Build history of the part. All positions in model axes, mm. A direction names the side the tool comes from. Give positions to 0.01 mm unless a question says otherwise; leave off trailing zeros. Order: outer loops, then holes, each group sorted by start corner. A loop starts at its lowest first (then second) coordinate and runs counter-clockwise, first axis right, second up. Notation, with made-up numbers: (-11.75, 78) -> (27.25, 78) arc R19 ccw to (27.25, 86) -> close; hole circle Ø2 at (8, 0.25). An arc over 180 degrees is marked (long way). One line per item, written item: value. Start each with the question number.
(1) Pin check, flat tip, straight feed: pin 1 (15 mm diameter, centred on x = -41.5, z = -49, fed in from +Y). Stop position of the tip, or through.
(2) Which spindle directions (+Z, -Z, +X, -X, +Y, -Y) get a long thin tool onto all of the face, cutting with end or side? Do faces 5 (the flat face through (16, 0, -18)), 6 (the cylindrical face through (-26.452, 14.93, -40.881)). Say none if no direction does.
(3) Saw through at C-C on x = 14.5. Give the cut face in (y, z).
(4) Saw through at A-A on y = 15.5. Give the cut face in (x, z).
(5) Probe line 1 (X direction, y = 16, z = -45); line 2 (X direction, y = 14, z = 0); line 3 (Z direction, x = 60.5, y = 13.5). List the from-to ranges inside material, lowest first.
(6) Two-plate mould, pull along X, no slides. Class faces 1 (the flat face through (-70, 10, -70)), 2 (the flat face through (75, 10, 1)), 3 (the flat face through (-1, 10, 28)), 4 (the flat face through (-68, 20, -1)): +X half, -X half, draft (parallel to the pull), parting line (faces both ways), or undercut.
(7) Saw through at B-B on z = -16. Give the cut face in (x, y), plus the area to 3 significant figures.
(8) Saw through at D-D on y = 4.5. Give the cut face in (x, z), plus the area to 3 significant figures.
```python
from build123d import *

# Parameters (mm, degrees)
SKETCH1_W           = 150
SKETCH1_H           = 150
SKETCH1_W_2         = 130
SKETCH1_H_2         = 130
BOSS_EXTRUDE2_DEPTH = 20
SKETCH1_4_W         = 130
SKETCH1_4_H         = 130
BOSS_EXTRUDE3_DEPTH = 10
CHAMFER1_SIZE       = 10
SKETCH2_R           = 20
CUT_EXTRUDE2_DEPTH  = 10
BOSS_EXTRUDE4_START = 10
SKETCH3_R           = 25
SKETCH3_R_2         = 20
BOSS_EXTRUDE4_DEPTH = 10
SKETCH4_R           = 19
SKETCH4_R_2         = 15
BOSS_EXTRUDE5_DEPTH = 10


with BuildPart() as part:
    # Sketch1 → Boss-Extrude2 (new body)
    with BuildSketch(Plane(origin=(0, 0, 0), x_dir=(1, 0, 0), z_dir=(0, 1, 0))):
        Rectangle(SKETCH1_W, SKETCH1_H)
        Rectangle(SKETCH1_W_2, SKETCH1_H_2, mode=Mode.SUBTRACT)
    extrude(amount=BOSS_EXTRUDE2_DEPTH)

    # Sketch1<4> → Boss-Extrude3 (add)
    with BuildSketch(Plane(origin=(0, 0, 0), x_dir=(1, 0, 0), z_dir=(0, 1, 0))):
        Rectangle(SKETCH1_4_W, SKETCH1_4_H)
    extrude(amount=BOSS_EXTRUDE3_DEPTH)

    # Chamfer1
    chamfer1_edges = [part.edges().sort_by_distance(p)[0] for p in [
        (75, 10, 75),
        (-75, 10, 75),
        (-75, 10, -75),
        (75, 10, -75),
    ]]
    chamfer(chamfer1_edges, length=CHAMFER1_SIZE)

    # Sketch2 → Cut-Extrude2 (cut)
    with BuildSketch(Plane(origin=(0, 10, 0), x_dir=(1, 0, 0), z_dir=(0, 1, 0))):
        with Locations(Location((0, 0, 0), (0, 0, 270))):
            Circle(SKETCH2_R)
    extrude(amount=-CUT_EXTRUDE2_DEPTH, mode=Mode.SUBTRACT)

    # Sketch3 → Boss-Extrude4 (add)
    with BuildSketch(Plane(origin=(0, 10, 0), x_dir=(1, 0, 0), z_dir=(0, 1, 0)).offset(BOSS_EXTRUDE4_START)):
        with Locations(Location((0, 0, 0), (0, 0, 270))):
            Circle(SKETCH3_R)
        with Locations(Location((0, 0, 0), (0, 0, 270))):
            Circle(SKETCH3_R_2, mode=Mode.SUBTRACT)
    extrude(amount=-BOSS_EXTRUDE4_DEPTH)

    # Sketch4 → Boss-Extrude5 (add)
    with BuildSketch(Plane(origin=(0, 10, 0), x_dir=(1, 0, 0), z_dir=(0, 1, 0))):
        with Locations(Location((-45, 45, 0), (0, 0, 90))):
            Circle(SKETCH4_R)
        with Locations(Location((-45, 45, 0), (0, 0, 90))):
            Circle(SKETCH4_R_2, mode=Mode.SUBTRACT)
    extrude(amount=BOSS_EXTRUDE5_DEPTH)


solid = part.part
```
Results below:
1. pin 1: stops at y = 10
2. face 5: +Z, -Z, +X, -X, -Y
2. face 6: +Y
3. outline: (0, -75) -> (20, -75) -> (20, -65) -> (10, -65) -> (10, -20.37) -> (20, -20.37) -> (20, -13.77) -> (0, -13.77) -> close; (0, 13.77) -> (20, 13.77) -> (20, 20.37) -> (10, 20.37) -> (10, 65) -> (20, 65) -> (20, 75) -> (0, 75) -> close
4. outline: (-75, -65) -> (-65, -75) -> (65, -75) -> (75, -65) -> (75, 65) -> (65, 75) -> (-65, 75) -> (-75, 65) -> close; circle Ø38 at (-45, -45); circle Ø50 at (0, 0); hole (-65, -65) -> (65, -65) -> (65, 65) -> (-65, 65) -> close; hole circle Ø30 at (-45, -45); hole circle Ø40 at (0, 0)
5. line 1: x = -75 to -65, -64 to -60, -30 to -26, 65 to 75
5. line 2: x = -75 to -65, -25 to -20, 20 to 25, 65 to 75
5. line 3: z = -75 to -65, 65 to 75
6. face 1: -X half
6. face 2: +X half
6. face 3: undercut
6. face 4: draft
7. outline: (-75, 0) -> (-12, 0) -> (-12, 20) -> (-19.21, 20) -> (-19.21, 10) -> (-65, 10) -> (-65, 20) -> (-75, 20) -> close; (12, 0) -> (75, 0) -> (75, 20) -> (65, 20) -> (65, 10) -> (19.21, 10) -> (19.21, 20) -> (12, 20) -> close
7. area: 1,600 mm²
8. outline: (-75, -65) -> (-65, -75) -> (65, -75) -> (75, -65) -> (75, 65) -> (65, 75) -> (-65, 75) -> (-75, 65) -> close; hole circle Ø40 at (0, 0)
8. area: 21,000 mm²
